Autodesk Inventor part; units mm, degrees
ref_plane "YZ Plane" through (0, 0, 0) normal (1, 0, 0) x (0, 1, 0)
ref_plane "XZ Plane" through (0, 0, 0) normal (0, 1, 0) x (-1, 0, 0)
ref_plane "XY Plane" through (0, 0, 0) normal (0, 0, 1) x (1, 0, 0)
sketch "Sketch1" plane through (0, 0, 0) normal (1, 0, 0) x (0, 1, 0)
  circle A0 centre (0, 0) radius 4
  dimension "d0" = 8
extrude "Extrusion1" add sketch "Sketch1" along normal blind 14.2
sketch "Sketch2" plane through (14.2, 0, 0) normal (1, 0, 0) x (0, 0, -1)
  circle A0 centre (0, 0) radius 4
hole "Hole1" at (14.2, 0, 0) direction (-1, 0, 0) diameter 3 end through all
chamfer "Chamfer1" distance 0.5 angle 45 4 edges at (0, -4, 0) (0, 0, 1.5) (14.2, 0, 1.5) (14.2, -4, 0)
properties part number "Rear Fan Spacer"
Can you work these out from the model? Positions are in its coordinate system, mm. Give positions to 0.01 mm unless a question says otherwise; leave off trailing zeros. Write each loop counter-clockwise with the first axis right and the second up, starting at its lowest first coordinate (ties: lowest second). Pieces come first, ordered by that corner, then holes. Notation, with made-up numbers: (-2.5, 46) - (1.5, 46) arc R19 ccw to (1.5, 53) - close; hole circle Ø7 at (62, 59). An arc over 180 degrees is marked (long way). Write item = value, one per line. Start each with the question number.
1. Thinking about a two-plate mould opening in Z: for faces 1 (the face through (14.2, 2, -2)), 2 (the face through (7.01, -0.07, 1.5)), 3 (the face through (7.008, -0.867, 3.905)), which applies, released by +Z, released by -Z, zero draft, split by the parting line, or undercut?
2. Please list where these lines run through material, in increasing order: line 1 (Z direction, x = 4.5, y = 0); line 2 (Y direction, x = 1.25, z = 0.5); line 3 (Z direction, x = 9, y = 1.25).
3. Imagine slicing it at C-C (x = 3). Please give me the cut outline in (y, z).
4. For pin 1 (2 mm diameter, centred on x = 1.5, y = -2, fed in from -Z); pin 2 (1.8 mm diameter, centred on y = 0, z = 0, fed in from +X); pin 3 (2 mm diameter, centred on x = 9.5, y = 1.5, fed in from +Z), each with a flat end and sliding along its axis, tell me the tip position at first contact or that it passes through.
5. Imagine slicing it at A-A (y = 0). Please give me the cut outline in (x, z).
Worked answers:
q1.face_1 = zero draft
q1.face_2 = undercut
q1.face_3 = split by the parting line
q2.line_1 = -4 to -1.5, 1.5 to 4
q2.line_2 = -3.97 to -1.41, 1.41 to 3.97
q2.line_3 = -3.8 to -0.83, 0.83 to 3.8
q3.outline = circle Ø8 at (0, 0); hole circle Ø3 at (0, 0)
q4.pin_1 = -3.87
q4.pin_2 = through
q4.pin_3 = 3.97
q5.outline = (0, -3.5) - (0.5, -4) - (13.7, -4) - (14.2, -3.5) - (14.2, -2) - (13.7, -1.5) - (0.5, -1.5) - (0, -2) - close; (0, 2) - (0.5, 1.5) - (13.7, 1.5) - (14.2, 2) - (14.2, 3.5) - (13.7, 4) - (0.5, 4) - (0, 3.5) - close
